For this review, take the finished solid that the model builds, in its own axes (mm). Face numbers are marked on the shaded views. Coordinates: 2 decimals unless noted, no trailing zeros. Loops run counter-clockwise (first coordinate to the right, second up) from the corner with the lowest first, then second, coordinate; pieces in that order, holes last. Notation, with made-up numbers: M 68.5,-9.5 L 94.5,-9.5 A7 cw 94.5,1.5 Z; hole C 18.25,85.25 d1. An arc over 180 degrees is marked long. Put each result on its own line as item: value.
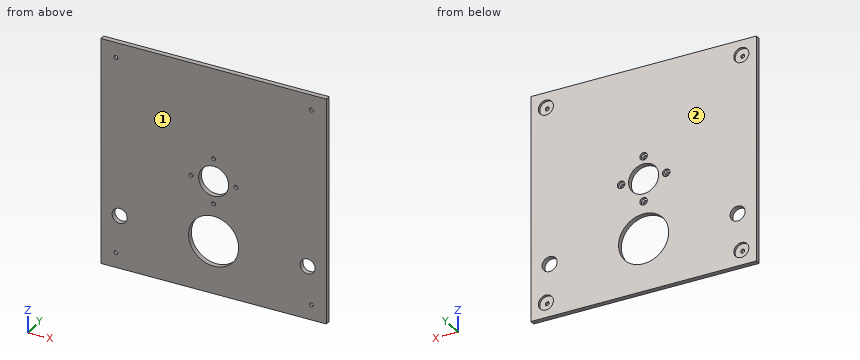
```python
from build123d import *

# Parameters (mm, degrees)
CROQUIS1_W              = 450
CROQUIS1_H              = 450
CROQUIS1_R              = 30
CROQUIS1_R_2            = 50
CROQUIS1_R_3            = 15
SALIENTE_EXTRUIR1_DEPTH = 10
CROQUIS7_R              = 15
CROQUIS7_R_2            = 7.5
CORTAR_EXTRUIR6_DEPTH   = 5
CROQUIS8_R              = 4
CORTAR_EXTRUIR7_DEPTH   = 5


with BuildPart() as part:
    # Croquis1 → Saliente-Extruir1 (new body)
    with BuildSketch(Plane(origin=(0, 0, 0), x_dir=(1, 0, 0), z_dir=(0, 1, 0))):
        Rectangle(CROQUIS1_W, CROQUIS1_H)
        Circle(CROQUIS1_R, mode=Mode.SUBTRACT)
        with Locations((0, 120)):
            Circle(CROQUIS1_R_2, mode=Mode.SUBTRACT)
        with Locations((-187.5, 120)):
            Circle(CROQUIS1_R_3, mode=Mode.SUBTRACT)
        with Locations((187.5, 120)):
            Circle(CROQUIS1_R_3, mode=Mode.SUBTRACT)
    extrude(amount=SALIENTE_EXTRUIR1_DEPTH)

    # Croquis7 → Cortar-Extruir6 (cut)
    with BuildSketch(Plane(origin=(0, 10, 0), x_dir=(1, 0, 0), z_dir=(0, 1, 0))):
        with Locations((-195, 195)):
            Circle(CROQUIS7_R)
        with Locations((195, 195)):
            Circle(CROQUIS7_R)
        with Locations((195, -195)):
            Circle(CROQUIS7_R)
        with Locations((-195, -195)):
            Circle(CROQUIS7_R)
        with Locations((-45, 0)):
            Circle(CROQUIS7_R_2)
        with Locations((0, 45)):
            Circle(CROQUIS7_R_2)
        with Locations((0, -45)):
            Circle(CROQUIS7_R_2)
        with Locations((45, 0)):
            Circle(CROQUIS7_R_2)
    extrude(amount=-CORTAR_EXTRUIR6_DEPTH, mode=Mode.SUBTRACT)

    # Croquis8 → Cortar-Extruir7 (cut)
    with BuildSketch(Plane(origin=(0, 5, 0), x_dir=(1, 0, 0), z_dir=(0, 1, 0))):
        with Locations((195, -195)):
            Circle(CROQUIS8_R)
        with Locations((-195, -195)):
            Circle(CROQUIS8_R)
        with Locations((-45, 0)):
            Circle(CROQUIS8_R)
        with Locations((45, 0)):
            Circle(CROQUIS8_R)
        with Locations((0, -45)):
            Circle(CROQUIS8_R)
        with Locations((0, 45)):
            Circle(CROQUIS8_R)
        with Locations((195, 195)):
            Circle(CROQUIS8_R)
        with Locations((-195, 195)):
            Circle(CROQUIS8_R)
    extrude(amount=-CORTAR_EXTRUIR7_DEPTH, mode=Mode.SUBTRACT)


solid = part.part
```
(1) For pin 1 (18 mm diameter, centred on x = 187.5, z = -120, fed in from -Y); pin 2 (10.5 mm diameter, centred on x = 0, z = 45, fed in from -Y); pin 3 (7.5 mm diameter, centred on x = -46.5, z = -1.5, fed in from +Y), all flat-tipped, find the tip position at first contact; note any pin that passes through.
Determined:
pin 1: passes through
pin 2: stops at y = 0
pin 3: stops at y = 5
(2) Add section B-B (y = 3.5). State how many separate pieces and enclosed holes the cut face has, plus the area to 3 significant figures.
Determined:
separate pieces: 1
enclosed holes: 12
area: 190,000 mm^2
(3) Add section A-A (z = -120). Write out the cut boundary in (x, y).
Determined:
outline: M -225,0 L -202.5,0 L -202.5,10 L -225,10 Z; M -172.5,0 L -50,0 L -50,10 L -172.5,10 Z; M 50,0 L 172.5,0 L 172.5,10 L 50,10 Z; M 202.5,0 L 225,0 L 225,10 L 202.5,10 Z
(4) Wall thickness on line 1 along X through (y, z) = (1.6, -195); line 2 along X through (y, z) = (7, -120); line 3 along X through (y, z) = (2.25, 45): over which ranges is each line inside the solid? List them lowest first. Write a range as [from, to].
Determined:
line 1: x = [-225, -199], [-191, 191], [199, 225]
line 2: x = [-225, -202.5], [-172.5, -50], [50, 172.5], [202.5, 225]
line 3: x = [-225, -4], [4, 225]
(5) Draft analysis for pull direction Y (two halves, no side actions). For the marked faces 1 and 2, state which applies: +Y half, -Y half, draft (parallel to the pull), parting line (faces both ways), or undercut.
Determined:
face 1: -Y half
face 2: +Y half
(6) Add section C-C (z = -20.5). Write out the cut boundary in (x, y), plus the area to 3 significant figures.
Determined:
outline: M -225,0 L -21.9,0 L -21.9,10 L -225,10 Z; M 21.9,0 L 225,0 L 225,10 L 21.9,10 Z
area: 4,060 mm^2
